```python
from build123d import *
from OCP.BRepFilletAPI import BRepFilletAPI_MakeChamfer

# Parameters (mm, degrees)
SKETCH1_W                   = 2.794
SKETCH1_H                   = 2.54
BOSS_EXTRUDE1_DEPTH         = 4.2545
SKETCH3_W                   = 0.4064
SKETCH3_H                   = 0.6096
CHAMFER1_SIZE               = 0.254
CHAMFER1_SIZE2              = 0.146646968
SKETCH4_W                   = 1.778
SKETCH4_H                   = 1.524
CUT_EXTRUDE1_DEPTH          = 6.35
CHAMFER2_SIZE               = 0.254
CHAMFER2_SIZE2              = 0.146646968
LPATTERN1_COUNT             = 4
LPATTERN1_PITCH             = 2.54
CHAMFER1_OF_LPATTERN1_SIZE  = 0.254
CHAMFER1_OF_LPATTERN1_SIZE2 = 0.146646968
CHAMFER2_OF_LPATTERN1_SIZE2 = 0.146646968
CHAMFER2_OF_LPATTERN1_SIZE  = 0.254


with BuildPart() as part:
    # Sketch1 → Boss-Extrude1 (new, symmetric)
    with BuildSketch(Plane.XY):
        Rectangle(SKETCH1_W, SKETCH1_H)
    boss_extrude1 = extrude(amount=BOSS_EXTRUDE1_DEPTH, both=True)

    # Sweep1: sweep along a path in Sketch2
    with BuildLine(Plane(origin=(0, 0, 0), x_dir=(0, 0, -1), z_dir=(1, 0, 0))) as sweep1_path:
        Line((5.8547, -4.4196), (5.8547, -1.6002))
        ThreePointArc((5.8547, -1.6002), (5.386012271, -0.468687729), (4.2545, 0))
    # Sketch3 → Sweep1 (sweep)
    with BuildSketch(Plane(origin=(0, 0, -4.2545), x_dir=(-1, 0, 0), z_dir=(0, 0, -1))):
        Rectangle(SKETCH3_W, SKETCH3_H)
    sweep1 = sweep(path=sweep1_path.line)

    # Chamfer1: one chamfer whose edges measure the first distance from different faces: ONE call of the kernel's chamfer builder (chamfer() names one face for all edges)
    chamfer1_edges_1 = [part.edges().sort_by_distance(p)[0] for p in [
        (-0.2032, -4.4196, -5.8547),
    ]]
    chamfer1_side_1 = [part.faces().sort_by_distance(p)[0] for p in [
        (-0.2032, -1.859510613, -5.586438348),
    ]]
    chamfer1_edges_2 = [part.edges().sort_by_distance(p)[0] for p in [
        (0, -4.4196, -6.1595),
    ]]
    chamfer1_side_2 = [part.faces().sort_by_distance(p)[0] for p in [
        (0, -3.0099, -6.1595),
    ]]
    chamfer1_edges_3 = [part.edges().sort_by_distance(p)[0] for p in [
        (0.2032, -4.4196, -5.8547),
    ]]
    chamfer1_side_3 = [part.faces().sort_by_distance(p)[0] for p in [
        (0.2032, -1.859510613, -5.586438348),
    ]]
    chamfer1_edges_4 = [part.edges().sort_by_distance(p)[0] for p in [
        (0, -4.4196, -5.5499),
    ]]
    chamfer1_side_4 = [part.faces().sort_by_distance(p)[0] for p in [
        (0, -3.0099, -5.5499),
    ]]
    chamfer1 = BRepFilletAPI_MakeChamfer(part.part.solid().wrapped)
    for e in chamfer1_edges_1:
        chamfer1.Add(CHAMFER1_SIZE, CHAMFER1_SIZE2, e.wrapped, chamfer1_side_1[0].wrapped)  # the first distance lies on this face
    for e in chamfer1_edges_2:
        chamfer1.Add(CHAMFER1_SIZE, CHAMFER1_SIZE2, e.wrapped, chamfer1_side_2[0].wrapped)  # the first distance lies on this face
    for e in chamfer1_edges_3:
        chamfer1.Add(CHAMFER1_SIZE, CHAMFER1_SIZE2, e.wrapped, chamfer1_side_3[0].wrapped)  # the first distance lies on this face
    for e in chamfer1_edges_4:
        chamfer1.Add(CHAMFER1_SIZE, CHAMFER1_SIZE2, e.wrapped, chamfer1_side_4[0].wrapped)  # the first distance lies on this face
    add(Compound.cast(chamfer1.Shape()), mode=Mode.REPLACE)

    # Sketch4 → Cut-Extrude1 (cut)
    with BuildSketch(Plane.XY.offset(4.2545)):
        Rectangle(SKETCH4_W, SKETCH4_H)
    cut_extrude1 = extrude(amount=-CUT_EXTRUDE1_DEPTH, mode=Mode.SUBTRACT)

    # Chamfer2
    chamfer2_edges = [part.edges().sort_by_distance(p)[0] for p in [
        (0.889, 0, 4.2545),
        (0, 0.762, 4.2545),
        (-0.889, 0, 4.2545),
        (0, -0.762, 4.2545),
    ]]
    chamfer2_side = [part.faces().sort_by_distance(p)[0] for p in [
        (0, -1.232240185, 4.2545),
    ]]
    chamfer(chamfer2_edges, length=CHAMFER2_SIZE, length2=CHAMFER2_SIZE2, reference=chamfer2_side[0])

    # LPattern1: Boss-Extrude1, Sweep1, Cut-Extrude1 ×4
    with Locations(*[(i * LPATTERN1_PITCH, 0, 0) for i in range(1, LPATTERN1_COUNT)]):
        add(boss_extrude1)
        add(sweep1)
        add(cut_extrude1, mode=Mode.SUBTRACT)

    # Chamfer1 of LPattern1: one chamfer whose edges measure the first distance from different faces: ONE call of the kernel's chamfer builder (chamfer() names one face for all edges)
    chamfer1_of_lpattern1_edges_1 = [part.edges().sort_by_distance(p)[0] for p in [
        (2.3368, -4.4196, -5.8547),
    ]]
    chamfer1_of_lpattern1_side_1 = [part.faces().sort_by_distance(p)[0] for p in [
        (2.3368, -1.859510613, -5.586438348),
    ]]
    chamfer1_of_lpattern1_edges_2 = [part.edges().sort_by_distance(p)[0] for p in [
        (2.54, -4.4196, -6.1595),
    ]]
    chamfer1_of_lpattern1_side_2 = [part.faces().sort_by_distance(p)[0] for p in [
        (2.54, -3.0099, -6.1595),
    ]]
    chamfer1_of_lpattern1_edges_3 = [part.edges().sort_by_distance(p)[0] for p in [
        (2.7432, -4.4196, -5.8547),
    ]]
    chamfer1_of_lpattern1_side_3 = [part.faces().sort_by_distance(p)[0] for p in [
        (2.7432, -1.859510613, -5.586438348),
    ]]
    chamfer1_of_lpattern1_edges_4 = [part.edges().sort_by_distance(p)[0] for p in [
        (2.54, -4.4196, -5.5499),
    ]]
    chamfer1_of_lpattern1_side_4 = [part.faces().sort_by_distance(p)[0] for p in [
        (2.54, -3.0099, -5.5499),
    ]]
    chamfer1_of_lpattern1_edges_5 = [part.edges().sort_by_distance(p)[0] for p in [
        (4.8768, -4.4196, -5.8547),
    ]]
    chamfer1_of_lpattern1_side_5 = [part.faces().sort_by_distance(p)[0] for p in [
        (4.8768, -1.859510613, -5.586438348),
    ]]
    chamfer1_of_lpattern1_edges_6 = [part.edges().sort_by_distance(p)[0] for p in [
        (5.08, -4.4196, -6.1595),
    ]]
    chamfer1_of_lpattern1_side_6 = [part.faces().sort_by_distance(p)[0] for p in [
        (5.08, -3.0099, -6.1595),
    ]]
    chamfer1_of_lpattern1_edges_7 = [part.edges().sort_by_distance(p)[0] for p in [
        (5.2832, -4.4196, -5.8547),
    ]]
    chamfer1_of_lpattern1_side_7 = [part.faces().sort_by_distance(p)[0] for p in [
        (5.2832, -1.859510613, -5.586438348),
    ]]
    chamfer1_of_lpattern1_edges_8 = [part.edges().sort_by_distance(p)[0] for p in [
        (5.08, -4.4196, -5.5499),
    ]]
    chamfer1_of_lpattern1_side_8 = [part.faces().sort_by_distance(p)[0] for p in [
        (5.08, -3.0099, -5.5499),
    ]]
    chamfer1_of_lpattern1_edges_9 = [part.edges().sort_by_distance(p)[0] for p in [
        (7.4168, -4.4196, -5.8547),
    ]]
    chamfer1_of_lpattern1_side_9 = [part.faces().sort_by_distance(p)[0] for p in [
        (7.4168, -1.859510613, -5.586438348),
    ]]
    chamfer1_of_lpattern1_edges_10 = [part.edges().sort_by_distance(p)[0] for p in [
        (7.62, -4.4196, -6.1595),
    ]]
    chamfer1_of_lpattern1_side_10 = [part.faces().sort_by_distance(p)[0] for p in [
        (7.62, -3.0099, -6.1595),
    ]]
    chamfer1_of_lpattern1_edges_11 = [part.edges().sort_by_distance(p)[0] for p in [
        (7.8232, -4.4196, -5.8547),
    ]]
    chamfer1_of_lpattern1_side_11 = [part.faces().sort_by_distance(p)[0] for p in [
        (7.8232, -1.859510613, -5.586438348),
    ]]
    chamfer1_of_lpattern1_edges_12 = [part.edges().sort_by_distance(p)[0] for p in [
        (7.62, -4.4196, -5.5499),
    ]]
    chamfer1_of_lpattern1_side_12 = [part.faces().sort_by_distance(p)[0] for p in [
        (7.62, -3.0099, -5.5499),
    ]]
    chamfer1_of_lpattern1 = BRepFilletAPI_MakeChamfer(part.part.solid().wrapped)
    for e in chamfer1_of_lpattern1_edges_1:
        chamfer1_of_lpattern1.Add(CHAMFER1_OF_LPATTERN1_SIZE, CHAMFER1_OF_LPATTERN1_SIZE2, e.wrapped, chamfer1_of_lpattern1_side_1[0].wrapped)  # the first distance lies on this face
    for e in chamfer1_of_lpattern1_edges_2:
        chamfer1_of_lpattern1.Add(CHAMFER1_OF_LPATTERN1_SIZE, CHAMFER1_OF_LPATTERN1_SIZE2, e.wrapped, chamfer1_of_lpattern1_side_2[0].wrapped)  # the first distance lies on this face
    for e in chamfer1_of_lpattern1_edges_3:
        chamfer1_of_lpattern1.Add(CHAMFER1_OF_LPATTERN1_SIZE, CHAMFER1_OF_LPATTERN1_SIZE2, e.wrapped, chamfer1_of_lpattern1_side_3[0].wrapped)  # the first distance lies on this face
    for e in chamfer1_of_lpattern1_edges_4:
        chamfer1_of_lpattern1.Add(CHAMFER1_OF_LPATTERN1_SIZE, CHAMFER1_OF_LPATTERN1_SIZE2, e.wrapped, chamfer1_of_lpattern1_side_4[0].wrapped)  # the first distance lies on this face
    for e in chamfer1_of_lpattern1_edges_5:
        chamfer1_of_lpattern1.Add(CHAMFER1_OF_LPATTERN1_SIZE, CHAMFER1_OF_LPATTERN1_SIZE2, e.wrapped, chamfer1_of_lpattern1_side_5[0].wrapped)  # the first distance lies on this face
    for e in chamfer1_of_lpattern1_edges_6:
        chamfer1_of_lpattern1.Add(CHAMFER1_OF_LPATTERN1_SIZE, CHAMFER1_OF_LPATTERN1_SIZE2, e.wrapped, chamfer1_of_lpattern1_side_6[0].wrapped)  # the first distance lies on this face
    for e in chamfer1_of_lpattern1_edges_7:
        chamfer1_of_lpattern1.Add(CHAMFER1_OF_LPATTERN1_SIZE, CHAMFER1_OF_LPATTERN1_SIZE2, e.wrapped, chamfer1_of_lpattern1_side_7[0].wrapped)  # the first distance lies on this face
    for e in chamfer1_of_lpattern1_edges_8:
        chamfer1_of_lpattern1.Add(CHAMFER1_OF_LPATTERN1_SIZE, CHAMFER1_OF_LPATTERN1_SIZE2, e.wrapped, chamfer1_of_lpattern1_side_8[0].wrapped)  # the first distance lies on this face
    for e in chamfer1_of_lpattern1_edges_9:
        chamfer1_of_lpattern1.Add(CHAMFER1_OF_LPATTERN1_SIZE, CHAMFER1_OF_LPATTERN1_SIZE2, e.wrapped, chamfer1_of_lpattern1_side_9[0].wrapped)  # the first distance lies on this face
    for e in chamfer1_of_lpattern1_edges_10:
        chamfer1_of_lpattern1.Add(CHAMFER1_OF_LPATTERN1_SIZE, CHAMFER1_OF_LPATTERN1_SIZE2, e.wrapped, chamfer1_of_lpattern1_side_10[0].wrapped)  # the first distance lies on this face
    for e in chamfer1_of_lpattern1_edges_11:
        chamfer1_of_lpattern1.Add(CHAMFER1_OF_LPATTERN1_SIZE, CHAMFER1_OF_LPATTERN1_SIZE2, e.wrapped, chamfer1_of_lpattern1_side_11[0].wrapped)  # the first distance lies on this face
    for e in chamfer1_of_lpattern1_edges_12:
        chamfer1_of_lpattern1.Add(CHAMFER1_OF_LPATTERN1_SIZE, CHAMFER1_OF_LPATTERN1_SIZE2, e.wrapped, chamfer1_of_lpattern1_side_12[0].wrapped)  # the first distance lies on this face
    add(Compound.cast(chamfer1_of_lpattern1.Shape()), mode=Mode.REPLACE)

    # Chamfer2 of LPattern1
    chamfer2_of_lpattern1_edges = [part.edges().sort_by_distance(p)[0] for p in [
        (3.429, 0, 4.2545),
        (2.54, 0.762, 4.2545),
        (1.651, 0, 4.2545),
        (2.54, -0.762, 4.2545),
        (5.969, 0, 4.2545),
        (5.08, 0.762, 4.2545),
        (4.191, 0, 4.2545),
        (5.08, -0.762, 4.2545),
        (8.509, 0, 4.2545),
        (7.62, 0.762, 4.2545),
        (6.731, 0, 4.2545),
        (7.62, -0.762, 4.2545),
    ]]
    chamfer(chamfer2_of_lpattern1_edges, length=CHAMFER2_OF_LPATTERN1_SIZE, length2=CHAMFER2_OF_LPATTERN1_SIZE2)


solid = part.part
```
Design review of the part built by this model. Coordinates are the model's own, in mm. A direction names the side the tool comes from. Coordinates: 2 decimals unless noted, no trailing zeros. Order: outer loops, then holes, each group sorted by start corner. A loop starts at its lowest first (then second) coordinate and runs counter-clockwise, first axis right, second up. Notation, with made-up numbers: (-13.75, 53.25) - (-7.75, 53.25) arc R21 cw to (-7.75, 79.25) - close; hole circle Ø8 at (47.5, 89.25). An arc over 180 degrees is marked (long way). Answer in a Markdown table with one row per item.
(1) For faces 1 (the cylindrical face through (2.537, -0.694, -5.181)), 2 (the flat face through (6.731, 0, 1)), 3 (the flat face through (4.877, -2, -6)), 4 (the flat face through (4, -1.27, 0)), list the 3-axis set-ups (+Z, -Z, +X, -X, +Y, -Y) from which the entire face can be reached by the end or side of a thin tool; tool diameter is ignored.
Checked values:
| item | result |
|---|---|
| face 1 | +X, -X, -Y |
| face 2 | +Z |
| face 3 | -Z, +Y, -Y |
| face 4 | +Z, +X, -X, -Y |
(2) Consider section C-C on x = 8. State the section outline as (y, z) points, plus the area to 3 significant figures.
Checked values:
| item | result |
|---|---|
| outline | (-1.27, -4.25) - (1.27, -4.25) - (1.27, 4.25) - (1.02, 4.25) - (0.76, 4.11) - (0.76, -2.1) - (-0.76, -2.1) - (-0.76, 4.11) - (-1.02, 4.25) - (-1.27, 4.25) - close |
| area | 11.9 mm^2 |
(3) Clearance check with flat-ended pins moving along their axes: pin 1 (2 mm diameter, centred on y = -1.5, z = -5.5, fed in from -X); pin 2 (5 mm diameter, centred on x = 3.5, z = 2, fed in from -Y); pin 3 (2 mm diameter, centred on x = 3.5, y = -0.5, fed in from -Z); pin 4 (1 mm diameter, centred on y = -2.5, z = -2.5, fed in from -X). State where each tip first meets the part, or that it passes through.
Checked values:
| item | result |
|---|---|
| pin 1 | x = -0.2 |
| pin 2 | y = -1.27 |
| pin 3 | z = -6.11 |
| pin 4 | through |
(4) Wall thickness on line 1 along X through (y, z) = (-0.4, 2.25); line 2 along Y through (x, z) = (3.25, 3.75); line 3 along Z through (x, y) = (0.25, -0.3): over which ranges is each line inside the solid? List them lowest first. Write a range as from..to.
Checked values:
| item | result |
|---|---|
| line 1 | -1.4..-0.89, 0.89..1.65, 3.43..4.19, 5.97..6.73, 8.51..9.02 |
| line 2 | -1.27..-0.76, 0.76..1.27 |
| line 3 | -4.25..-2.1 |
(5) Consider section A-A on y = -2.05. State the section outline as (x, z) points, plus the area to 3 significant figures.
Checked values:
| item | result |
|---|---|
| outline | (-0.2, -6.16) - (0.2, -6.16) - (0.2, -5.55) - (-0.2, -5.55) - close; (2.34, -6.16) - (2.74, -6.16) - (2.74, -5.55) - (2.34, -5.55) - close; (4.88, -6.16) - (5.28, -6.16) - (5.28, -5.55) - (4.88, -5.55) - close; (7.42, -6.16) - (7.82, -6.16) - (7.82, -5.55) - (7.42, -5.55) - close |
| area | 0.991 mm^2 |
(6) The part is to be moulded in two halves that separate along X. For faces 5 (the cylindrical face through (-0.003, -0.694, -5.181)), 6 (the flat face through (-1.397, 0, 0)), 7 (the flat face through (2.743, -2, -6)), 8 (the flat face through (9.017, 0, 0)), say which applies: released by +X, released by -X, zero draft, split by the parting line, or undercut.
Checked values:
| item | result |
|---|---|
| face 5 | zero draft |
| face 6 | released by -X |
| face 7 | undercut |
| face 8 | released by +X |
(7) Consider section D-D on z = -3. State the section outline as (x, y) points.
Checked values:
| item | result |
|---|---|
| outline | (-1.4, -1.27) - (9.02, -1.27) - (9.02, 1.27) - (-1.4, 1.27) - close |
(8) Consider section B-B on z = 0. State the section outline as (x, y) points, plus the area to 3 significant figures.
Checked values:
| item | result |
|---|---|
| outline | (-1.4, -1.27) - (9.02, -1.27) - (9.02, 1.27) - (-1.4, 1.27) - close; hole (-0.89, -0.76) - (0.89, -0.76) - (0.89, 0.76) - (-0.89, 0.76) - close; hole (1.65, -0.76) - (3.43, -0.76) - (3.43, 0.76) - (1.65, 0.76) - close; hole (4.19, -0.76) - (5.97, -0.76) - (5.97, 0.76) - (4.19, 0.76) - close; hole (6.73, -0.76) - (8.51, -0.76) - (8.51, 0.76) - (6.73, 0.76) - close |
| area | 15.6 mm^2 |
